```python
from build123d import *

# Parameters (mm, degrees)
F0_W      = 100
F0_H      = 75
F1_DEPTH  = 40
F3_DEPTH  = 100.001
F4_W      = 60
F4_H      = 40
F5_DEPTH  = 35
F6_W      = 60
F6_H      = 10
F7_DEPTH  = 30
F8_W      = 20
F8_H      = 50
F9_DEPTH  = 20
F10_W     = 14
F10_H     = 47
F11_DEPTH = 17
F12_R     = 3
F13_R     = 6
F14_W     = 60
F14_H     = 75
F15_DEPTH = 15
F16_R     = 5
F17_DEPTH = 20


with BuildPart() as f1:
    # F0 (on Front) → F1 (new body)
    with BuildSketch(Plane.XZ):
        with Locations((50, 37.5)):
            Rectangle(F0_W, F0_H)
    extrude(amount=-F1_DEPTH)

    # F2 (on face) → F3 (cut, through all)
    with BuildSketch(Plane.YZ.offset(100)):
        Polygon((0, 0), (40, 75), (0, 75), align=None)
    extrude(amount=-F3_DEPTH, mode=Mode.SUBTRACT)

    # F4 (on Front) → F5 (cut)
    with BuildSketch(Plane.XZ):
        with Locations((50, 40)):
            Rectangle(F4_W, F4_H)
    extrude(amount=-F5_DEPTH, mode=Mode.SUBTRACT)

    # F6 (on face) → F7 (join)
    with BuildSketch(Plane.YZ.offset(100)):
        with Locations((70, 5)):
            Rectangle(F6_W, F6_H)
    extrude(amount=-F7_DEPTH)

    # F8 (on face) → F9 (join)
    with BuildSketch(Plane.XY.offset(10)):
        with Locations((85, 65)):
            Rectangle(F8_W, F8_H)
    extrude(amount=F9_DEPTH)

    # F10 (on face) → F11 (cut)
    with BuildSketch(Plane.XY.offset(30)):
        with Locations((85, 63.5)):
            Rectangle(F10_W, F10_H)
    extrude(amount=-F11_DEPTH, mode=Mode.SUBTRACT)

    # F12
    f12_edges = [f1.edges().sort_by_distance(p)[0] for p in [
        (78, 87, 21.5),
        (92, 87, 21.5),
    ]]
    fillet(f12_edges, radius=F12_R)

    # F13
    f13_edges = [f1.edges().sort_by_distance(p)[0] for p in [
        (75, 90, 20),
        (95, 90, 20),
    ]]
    fillet(f13_edges, radius=F13_R)

    # F14 (on face) → F15 (join)
    with BuildSketch(Plane(origin=(0, 0, 0), x_dir=(0, -1, 0), z_dir=(-1, 0, 0))):
        with Locations((-70, 37.5)):
            Rectangle(F14_W, F14_H)
    extrude(amount=-F15_DEPTH)

    # F16 (on face) → F17 (join)
    with BuildSketch(Plane.XY.offset(75)):
        with Locations((7, 60)):
            Circle(F16_R)
    extrude(amount=F17_DEPTH)


solid = f1.part
```
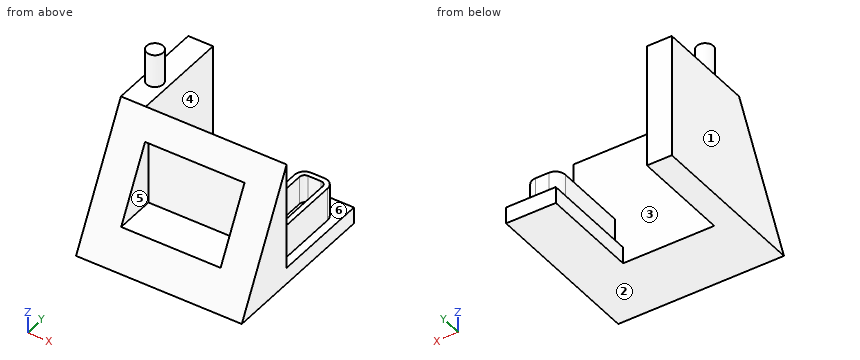
The listing builds one solid part. Answer for the finished solid, in the listing's coordinates (mm). Face numbers are marked on the shaded views. A direction names the side the tool comes from. Give positions to 0.01 mm unless a question says otherwise; leave off trailing zeros. Order: outer loops, then holes, each group sorted by start corner. A loop starts at its lowest first (then second) coordinate and runs counter-clockwise, first axis right, second up.
1) Find section A-A on y = 60. Write down the section's boundary in (x, z), then the cut area to 3 significant figures.
Reported:
outline: (0, 0) - (15, 0) - (15, 75) - (12, 75) - (12, 95) - (2, 95) - (2, 75) - (0, 75) - close; (70, 0) - (100, 0) - (100, 10) - (95, 10) - (95, 30) - (92, 30) - (92, 13) - (78, 13) - (78, 30) - (75, 30) - (75, 10) - (70, 10) - close
area: 1,790 mm2
2) Find section B-B on x = 41. Write down the section's boundary in (y, z).
Reported:
outline: (0, 0) - (40, 0) - (40, 75) - (32, 60) - (35, 60) - (35, 20) - (10.67, 20) - close
3) Find section C-C on y = 22. Write down the section's boundary in (x, z), then the cut area to 3 significant figures.
Reported:
outline: (0, 0) - (100, 0) - (100, 41.25) - (80, 41.25) - (80, 20) - (20, 20) - (20, 41.25) - (0, 41.25) - close
area: 2,850 mm2
4) Find section D-D on z = 63. Write down the section's boundary in (x, y).
Reported:
outline: (0, 33.6) - (100, 33.6) - (100, 40) - (15, 40) - (15, 100) - (0, 100) - close
5) Consider line 1 along X through (y, z) = (47, 4.5); line 2 along X through (y, z) = (15, 24); line 3 along X through (y, z) = (77, 48.5). Determine where each line is inside the solid, lowest interval first.
Reported:
line 1: x = 0 to 15, 70 to 100
line 2: x = 0 to 20, 80 to 100
line 3: x = 0 to 15
6) For the marked faces 4, 5 and 6, determine the directions among +Z, -Z, +X, -X, +Y, -Y from which every point of the face is accessible in a straight line to the end or side of a thin tool.
Reported:
face 4: +Z, -Z, +Y
face 5: -Y
face 6: +Z, +Y
7) Given P1, Ø4, axis at x = 88, z = 70, coming from the -Y side; P2, Ø4, axis at x = 86.5, z = 22.5, coming from the +Y side; P3, Ø1.5, axis at x = 48, y = 16.5, coming from the +Z side, each flat-ended and moving along its own axis, determine where each tip first touches the part or whether it passes through.
Reported:
P1: stops at y = 36.27
P2: stops at y = 90
P3: stops at z = 20
8) Determine the mould class of the marked faces 1, 2 and 3 for opening direction X: pulls with the +X half, pulls with the -X half, needs draft (parallel to the pull), parting line crosses it, or undercut.
Reported:
face 1: pulls with the -X half
face 2: needs draft
face 3: undercut
